```python
from build123d import *

# Parameters (mm, degrees)
SKETCH1_W           = 71
SKETCH1_H           = 34
SKETCH1_R           = 5
BOSS_EXTRUDE1_DEPTH = 8
SKETCH1_3_W         = 7
SKETCH1_3_H         = 34
BOSS_EXTRUDE2_DEPTH = 33
BOSS_EXTRUDE3_DEPTH = 80
CUT_EXTRUDE1_DEPTH  = 80
BOSS_EXTRUDE4_DEPTH = 7
CHAMFER1_SIZE2      = 34
CHAMFER1_SIZE       = 25


with BuildPart() as part:
    # Sketch1 → Boss-Extrude1 (new body)
    with BuildSketch(Plane(origin=(0, 0, 0), x_dir=(1, 0, 0), z_dir=(0, 1, 0))):
        with Locations((42.5, 17)):
            Rectangle(SKETCH1_W, SKETCH1_H)
        with Locations(Location((20, 17.695066584, 0), (0, 0, 270))):
            Circle(SKETCH1_R, mode=Mode.SUBTRACT)
        with Locations(Location((58, 17.695066584, 0), (0, 0, 270))):
            Circle(SKETCH1_R, mode=Mode.SUBTRACT)
    extrude(amount=BOSS_EXTRUDE1_DEPTH)

    # Sketch1<3> → Boss-Extrude2 (add)
    with BuildSketch(Plane(origin=(0, 0, 0), x_dir=(1, 0, 0), z_dir=(0, 1, 0))):
        with Locations((3.5, 17)):
            Rectangle(SKETCH1_3_W, SKETCH1_3_H)
    extrude(amount=BOSS_EXTRUDE2_DEPTH)

    # Sketch1<4> → Boss-Extrude3 (add)
    with BuildSketch(Plane(origin=(0, 0, 0), x_dir=(1, 0, 0), z_dir=(0, 1, 0))):
        Polygon((0, 41), (0, 34), (7, 34), (78, 34), (78, 41), align=None)
    extrude(amount=BOSS_EXTRUDE3_DEPTH)

    # Sketch2 → Cut-Extrude1 (cut)
    with BuildSketch(Plane.XY.offset(-34)):
        Polygon((0, 69.371997336), (78, 33), (78, 80), (0, 80), align=None)
    extrude(amount=-CUT_EXTRUDE1_DEPTH, mode=Mode.SUBTRACT)

    # Sketch3 → Boss-Extrude4 (add)
    with BuildSketch(Plane(origin=(26.571016534, 56.981728841, 0), x_dir=(0.9063077870366528, -0.42261826174069356, 0), z_dir=(0.42261826174069356, 0.9063077870366528, 0))):
        with BuildLine():
            Line((-19.317872928, 79), (-19.317872928, 60))
            Line((-19.317872928, 60), (-7.254395249, 60))
            ThreePointArc((-7.254395249, 60), (-6.082822373, 62.828427125), (-3.254395249, 64))
            Line((-3.254395249, 64), (18.683347003, 64))
            ThreePointArc((18.683347003, 64), (28.799829698, 68.762428879), (35.745604751, 60))
            Line((35.745604751, 60), (46.745604751, 60))
            Line((46.745604751, 60), (46.745604751, 79))
            Line((46.745604751, 79), (-19.317872928, 79))
        make_face()
        with BuildLine():
            Line((-19.317872928, 60), (-19.317872928, 41))
            Line((-19.317872928, 41), (46.745604751, 41))
            Line((46.745604751, 41), (46.745604751, 60))
            Line((46.745604751, 60), (35.745604751, 60))
            ThreePointArc((35.745604751, 60), (28.799829698, 51.237571121), (18.683347003, 56))
            Line((18.683347003, 56), (-3.254395249, 56))
            ThreePointArc((-3.254395249, 56), (-6.082822373, 57.171572875), (-7.254395249, 60))
            Line((-7.254395249, 60), (-19.317872928, 60))
        make_face()
    extrude(amount=-BOSS_EXTRUDE4_DEPTH)

    # Chamfer1
    chamfer1_edges = [part.edges().sort_by_distance(p)[0] for p in [
        (3.5, 33, 0),
    ]]
    chamfer1_side = [part.faces().sort_by_distance(p)[0] for p in [
        (3.5, 32.5, 0),
    ]]
    chamfer(chamfer1_edges, length=CHAMFER1_SIZE - 0.0001, length2=CHAMFER1_SIZE2 - 0.0001, reference=chamfer1_side[0])  # a hair under: the kernel refuses the full size


solid = part.part
```
Geometry check sheet. Reference: the model listing, model coordinates, mm. A direction names the side the tool comes from. Coordinates: 2 decimals unless noted, no trailing zeros. Order: outer loops, then holes, each group sorted by start corner. A loop starts at its lowest first (then second) coordinate and runs counter-clockwise, first axis right, second up.
Q1. Sectioned sample at B-B on x = 34. Record the cut outline in (y, z).
Reply:
outline: (0, -41) - (45.79, -41) - (45.79, -56) - (53.52, -56) - (53.52, -34) - (8, -34) - (8, 0) - (0, 0) - close; (45.79, -79) - (53.52, -79) - (53.52, -64) - (45.79, -64) - close
Q2. Thickness scan on probe 1 along Y at (x, z) = (57.5, -26); probe 2 along Z at (x, y) = (65, 21); probe 3 along Z at (x, y) = (13, 61). Record the ranges inside material, lowest first.
Reply:
probe 1: y = 0 to 8
probe 2: z = -41 to -34
probe 3: z = -79 to -34
Q3. Tool access check on faces 1 (the face through (67.48, 34.1, -59.73)), 2 (the face through (7, 18, -21)), 3 (the face through (7.605, 62.018, -60.266)). Record the directions out of +Z, -Z, +X, -X, +Y, -Y that give a thin tool (end or side, any length) a straight path to the whole face; none if there is none.
Reply:
face 1: -Z, +X, -Y
face 2: +Z, +X, +Y
face 3: -Z, -X, +Y
Q4. Depth check by flat-ended pin: pin 1 Ø1.5 at (y, z) = (61, -54.5) entering from -X; pin 2 Ø4 at (x, y) = (60, 37.5) entering from +Z; pin 3 Ø6 at (x, z) = (22, -41) entering from +Y. Enter the tip coordinate at first touch or a pass-through.
Reply:
pin 1: stops at x = 6.78
pin 2: stops at z = -34
pin 3: stops at y = 60.51
Q5. Sectioned sample at C-C on y = 20.5. Record the cut outline in (x, z).
Reply:
outline: (0, -41) - (78, -41) - (78, -34) - (7, -34) - (7, -17) - (0, -17) - close
Q6. Sectioned sample at A-A on z = -54. Record the cut outline in (x, y), and give its area (3 significant figures).
Reply:
outline: (6.1, 58.8) - (41.77, 42.17) - (44.73, 48.51) - (9.06, 65.15) - close; (53.93, 36.5) - (65.98, 30.88) - (68.94, 37.23) - (56.89, 42.84) - close
area: 369 mm2
Q7. Sectioned sample at D-D on z = -62. Record the cut outline in (x, y), and give its area (3 significant figures).
Reply:
outline: (6.1, 58.8) - (17.52, 53.48) - (20.48, 59.82) - (9.06, 65.15) - close; (55.81, 35.63) - (65.98, 30.88) - (68.94, 37.23) - (58.76, 41.97) - close
area: 167 mm2
Q8. Draft check along Z on faces 4 (the face through (3.451, 20.675, -17.238)), 5 (the face through (42, 8, -17)), 6 (the face through (32, 51, -56)). Enter one of: released by +Z, released by -Z, zero draft, split by the parting line, or undercut.
Reply:
face 4: released by +Z
face 5: zero draft
face 6: undercut
